Source: CAD feature listing. Evaluate the final solid. Frame: model axes, mm. Face numbers are marked on the shaded views. A direction names the side the tool comes from. Round coordinates to 2 decimals unless told otherwise and drop trailing zeros. Order: outer loops, then holes, each group sorted by start corner. A loop starts at its lowest first (then second) coordinate and runs counter-clockwise, first axis right, second up. Notation, with made-up numbers: (-31, 7.25) - (-22, 7.25) arc R17 cw to (-22, 38.25) - close; hole circle Ø9 at (46, -33). An arc over 180 degrees is marked (long way). Use one line per item in the form item = value. Start each with the question number.
Q1. Ray query, line 1 (X direction, y = -20.5, z = 13.5); line 2 (X direction, y = -15, z = 7). Return the intervals inside material, ascending. Write a range as [from, to].
Q2. Pin query (flat end, axial travel): pin 1 Ø4 at (y, z) = (-12, 16.5) entering from +X; pin 2 Ø10 at (y, z) = (-11.5, 14.5) entering from -X. Return the tip coordinate at first contact, or that it passes through.
Q3. Set-up query: the marked faces 1, 2 and 3. Return all of +Z, -Z, +X, -X, +Y, -Y with unobstructed straight access to the full face (end or side cutting, diameter ignored); none if empty.
Q4. Cut plane A-A, the plane y = -23. Return the cut outline in (x, z).
Q5. Cut plane B-B, the plane z = 12.5. Return the cut outline in (x, y).
from build123d import *

# Parameters (mm, degrees)
F0_W      = 88.9
F0_H      = 31.75
F1_DEPTH  = 25.4
F2_R      = 5.08
F1_FACE_W = 78.74
F1_FACE_H = 25.4
F3_DEPTH  = 12.7


with BuildPart() as f1:
    # F0 (on Front) → F1 (new body)
    with BuildSketch(Plane.XZ):
        with Locations((-44.45, -5.363265)):
            Rectangle(F0_W, F0_H)
    extrude(amount=F1_DEPTH)

    # F2
    f2_edges = [f1.edges().sort_by_distance(p)[0] for p in [
        (-88.9, -12.7, 10.511735),
        (0, -12.7, 10.511735),
    ]]
    fillet(f2_edges, radius=F2_R)

    # F1_face (on face) → F3 (join)
    with BuildSketch(Plane(origin=(-44.45, -12.7, 10.511735), x_dir=(1, 0, 0), z_dir=(0, 0, 1))):
        Rectangle(F1_FACE_W, F1_FACE_H)
    extrude(amount=F3_DEPTH)


solid = f1.part
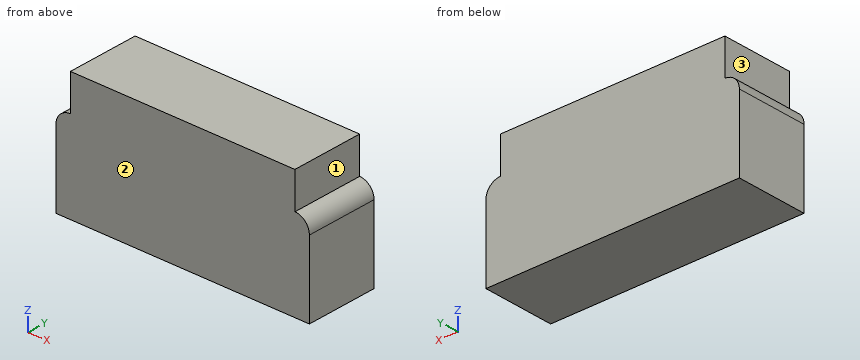
Completed:
q1.line_1 = [-83.82, -5.08]
q1.line_2 = [-88.65, -0.25]
q2.pin_1 = -5.08
q2.pin_2 = -86.86
q3.face_1 = +Z, +X, +Y, -Y
q3.face_2 = +Z, -Z, +X, -X, -Y
q3.face_3 = +Z, -X, +Y, -Y
q4.outline = (-88.9, -21.24) - (0, -21.24) - (0, 5.43) arc R5.08 ccw to (-5.08, 10.51) - (-5.08, 23.21) - (-83.82, 23.21) - (-83.82, 10.51) arc R5.08 ccw to (-88.9, 5.43) - close
q5.outline = (-83.82, -25.4) - (-5.08, -25.4) - (-5.08, 0) - (-83.82, 0) - close
